Here's how the part is built. I have some questions about the finished solid (model axes, mm). A direction names the side the tool comes from. Round coordinates to 2 decimals unless told otherwise and drop trailing zeros. Write each loop counter-clockwise with the first axis right and the second up, starting at its lowest first coordinate (ties: lowest second). Pieces come first, ordered by that corner, then holes. Notation, with made-up numbers: (-10.5, -10.5) -> (32.5, -10.5) arc R16 cw to (32.5, -3.5) -> close; hole circle Ø6 at (16, 36.25). An arc over 180 degrees is marked (long way). Answer in a Markdown table with one row per item.
from build123d import *

# Parameters (mm, degrees)
F1_DEPTH     = 38.1
F3_DEPTH     = 38.1
F5_D         = 6.35
F6_T1_DEPTH  = 20.7437886812
F6_T3_DEPTH  = 27.94
F6_T5_DEPTH  = 49.7055689591
F6_T7_DEPTH  = 20.4179452734
F6_T9_DEPTH  = 49.0300859467
F6_T11_DEPTH = 71.8058781858
F6_T13_DEPTH = 25.3882661408
F6_T15_DEPTH = 70.8375780274
F6_T17_DEPTH = 26.1528668654
F6_T22_DEPTH = 5.08
F6_T28_DEPTH = 5.08
F6_T34_DEPTH = 5.08
F6_T40_DEPTH = 5.08


# Not quite as in the source:
# - a fillet or chamfer that OpenCascade refuses, or shapes differently, is made with other operations: its cross-section is extruded or revolved along the edge and cut away or added


with BuildPart() as f1:
    # F0 (on Front) → F1 (new body)
    with BuildSketch(Plane.XZ):
        Polygon((0, 38.1), (0, 0.2683098665), (38.1, 0), (38.1, 38.1), align=None)
    extrude(amount=F1_DEPTH)

    # F2 (on face) → F3 (cut)
    with BuildSketch(Plane.XZ.offset(38.1)):
        Polygon((29.289287496, 38.1), (6.7755630988, 38.1), (19.05, 25.849385187), align=None)
        Polygon((0, 38.1), (0, 25.849385187), (6.7755630988, 38.1), align=None)
        Polygon((29.289287496, 38.1), (38.1, 25.849385187), (38.1, 38.1), align=None)
        Polygon((0, 0.2683098665), (18.8937886297, 0.1352550134), (0, 16.4943691343), align=None)
        Polygon((38.1, 16.4943691343), (20.8069253196, 0.1217822194), (38.1, 0), align=None)
    extrude(amount=-F3_DEPTH, mode=Mode.SUBTRACT)

    # F5 (through all)
    with Locations(Plane.YZ.offset(38.1)):
        with Locations((-19.05, 21.1718771607)):
            Hole(F5_D / 2)

    # F6: fillet of radius 5.08 on 16 edges, made by hand

    # F6_s2 → F6_t1 (cut)
    with BuildSketch(Plane.XY.offset(3.7943691343)):
        with BuildLine():
            ThreePointArc((5.08, 0), (1.4878975516, -1.4878975516), (0, -5.08))
            Line((0, -5.08), (0, 0))
            Line((0, 0), (5.08, 0))
        make_face()
        with BuildLine():
            ThreePointArc((5.08, -38.1), (1.4878975516, -36.6121024484), (0, -33.02))
            Line((0, -33.02), (0, -38.1))
            Line((0, -38.1), (5.08, -38.1))
        make_face()
    extrude(amount=F6_T1_DEPTH, mode=Mode.SUBTRACT)

    # F6_s4 → F6_t3 (cut)
    with BuildSketch(Plane.XZ.offset(5.08)):
        with BuildLine():
            ThreePointArc((0.634616087, 26.9968082311), (0.1612120254, 25.8077738444), (0, 24.5381578155))
            Line((0, 24.5381578155), (0, 25.849385187))
            Line((0, 25.849385187), (0.634616087, 26.9968082311))
        make_face()
        with BuildLine():
            ThreePointArc((37.1441471446, 27.1784247107), (37.8551353391, 25.7704755844), (38.1, 24.2123144077))
            Line((38.1, 24.2123144077), (38.1, 25.849385187))
            Line((38.1, 25.849385187), (37.1441471446, 27.1784247107))
        make_face()
    extrude(amount=F6_T3_DEPTH, mode=Mode.SUBTRACT)

    # F6_s6 → F6_t5 (cut)
    with BuildSketch(Plane.XZ.offset(-5.8027844796)):
        with BuildLine():
            ThreePointArc((1.754752754, 14.9750232202), (0.4594666969, 16.704305057), (0, 18.8154829261))
            Line((0, 18.8154829261), (0, 16.4943691343))
            Line((0, 16.4943691343), (1.754752754, 14.9750232202))
        make_face()
    extrude(amount=F6_T5_DEPTH, mode=Mode.SUBTRACT)

    # F6_s8 → F6_t7 (cut)
    with BuildSketch(Plane.XY.offset(3.7943691343)):
        with BuildLine():
            ThreePointArc((33.02, 0), (36.6121024484, -1.4878975516), (38.1, -5.08))
            Line((38.1, -5.08), (38.1, 0))
            Line((38.1, 0), (33.02, 0))
        make_face()
        with BuildLine():
            ThreePointArc((33.02, -38.1), (36.6121024484, -36.6121024484), (38.1, -33.02))
            Line((38.1, -33.02), (38.1, -38.1))
            Line((38.1, -38.1), (33.02, -38.1))
        make_face()
    extrude(amount=F6_T7_DEPTH, mode=Mode.SUBTRACT)

    # F6_s10 → F6_t9 (cut)
    with BuildSketch(Plane.XZ.offset(-5.4650429733)):
        with BuildLine():
            ThreePointArc((38.1, 18.6803863236), (37.6863002203, 16.6723917386), (36.5125817899, 14.991447121))
            Line((36.5125817899, 14.991447121), (38.1, 16.4943691343))
            Line((38.1, 16.4943691343), (38.1, 18.6803863236))
        make_face()
    extrude(amount=F6_T9_DEPTH, mode=Mode.SUBTRACT)

    # F6_s12 → F6_t11 (cut)
    with BuildSketch(Plane.XZ.offset(-16.8529390929)):
        with BuildLine():
            ThreePointArc((11.5469219559, 33.3379013421), (7.2465010014, 34.7721948924), (3.5129264291, 32.2009618637))
            Line((3.5129264291, 32.2009618637), (6.7755630988, 38.1))
            Line((6.7755630988, 38.1), (11.5469219559, 33.3379013421))
        make_face()
    extrude(amount=F6_T11_DEPTH, mode=Mode.SUBTRACT)

    # F6_s14 → F6_t13 (cut)
    with BuildSketch(Plane(origin=(11.5824663758, 0, 20.9417773971), x_dir=(0, 1, 0), z_dir=(0.4839863023, 0, 0.8750755734))):
        with BuildLine():
            ThreePointArc((-38.1, 7.4307483528), (-36.6121024484, 11.0228508012), (-33.02, 12.5107483528))
            Line((-33.02, 12.5107483528), (-38.1, 12.5107483528))
            Line((-38.1, 12.5107483528), (-38.1, 7.4307483528))
        make_face()
        with BuildLine():
            ThreePointArc((0, 7.4307483528), (-1.4878975516, 11.0228508012), (-5.08, 12.5107483528))
            Line((-5.08, 12.5107483528), (0, 12.5107483528))
            Line((0, 12.5107483528), (0, 7.4307483528))
        make_face()
    extrude(amount=F6_T13_DEPTH, mode=Mode.SUBTRACT)

    # F6_s16 → F6_t15 (cut)
    with BuildSketch(Plane.XZ.offset(-16.3687890137)):
        with BuildLine():
            ThreePointArc((25.0903071925, 33.076204123), (29.1727291737, 34.8949986115), (33.1122507828, 32.7844650022))
            Line((33.1122507828, 32.7844650022), (29.289287496, 38.1))
            Line((29.289287496, 38.1), (25.0903071925, 33.076204123))
        make_face()
    extrude(amount=F6_T15_DEPTH, mode=Mode.SUBTRACT)

    # F6_s18 → F6_t17 (cut)
    with BuildSketch(Plane(origin=(-15.4901461094, 0, 21.5378510306), x_dir=(0, 1, 0), z_dir=(0.5838799809, 0, -0.8118399891))):
        with BuildLine():
            ThreePointArc((-33.02, 46.024042114), (-36.6121024484, 44.5361445625), (-38.1, 40.944042114))
            Line((-38.1, 40.944042114), (-38.1, 46.024042114))
            Line((-38.1, 46.024042114), (-33.02, 46.024042114))
        make_face()
        with BuildLine():
            ThreePointArc((-5.08, 46.024042114), (-1.4878975516, 44.5361445625), (0, 40.944042114))
            Line((0, 40.944042114), (0, 46.024042114))
            Line((0, 46.024042114), (-5.08, 46.024042114))
        make_face()
    extrude(amount=F6_T17_DEPTH, mode=Mode.SUBTRACT)


with BuildPart() as f6_tool20:
    # F6_s21 → F6_t22 (new body)
    with BuildSketch(Plane.XZ.offset(5.08)):
        Polygon((5.08, 24.5381578155), (0.634616087, 26.9968082311), (0, 25.849385187), (0, 24.5381578155), align=None)
    extrude(amount=-F6_T22_DEPTH)

    # F6_s23 → F6_t24 (revolve, cut)
    with BuildSketch(Plane(origin=(5.08, -5.08, 24.5381578155), x_dir=(0.9682653493, 0, -0.2499244151), z_dir=(0.2499244151, 0, 0.9682653493))):
        with BuildLine():
            ThreePointArc((0, -5.08), (5.08, 0), (0, 5.08))
            Line((0, 5.08), (0, -5.08))
        make_face()
    revolve(axis=Axis((5.08, -5.08, 24.5381578155), (0, 1, 0)), mode=Mode.SUBTRACT)


with BuildPart() as f1_1:
    add(f1.part)

    # F6_t19: cut F6_tool20
    add(f6_tool20.part, mode=Mode.SUBTRACT)


with BuildPart() as f6_tool26:
    # F6_s27 → F6_t28 (new body)
    with BuildSketch(Plane.XZ.offset(33.02)):
        Polygon((5.08, 24.5381578155), (0.634616087, 26.9968082311), (0, 25.849385187), (0, 24.5381578155), align=None)
    extrude(amount=F6_T28_DEPTH)

    # F6_s29 → F6_t30 (revolve, cut)
    with BuildSketch(Plane(origin=(5.08, -33.02, 24.5381578155), x_dir=(0.9682653493, 0, -0.2499244151), z_dir=(-0.2499244151, 0, -0.9682653493))):
        with BuildLine():
            ThreePointArc((0, -5.08), (5.08, 0), (0, 5.08))
            Line((0, 5.08), (0, -5.08))
        make_face()
    revolve(axis=Axis((5.08, -33.02, 24.5381578155), (0, -1, 0)), mode=Mode.SUBTRACT)


with BuildPart() as f1_2:
    add(f1_1.part)

    # F6_t25: cut F6_tool26
    add(f6_tool26.part, mode=Mode.SUBTRACT)


with BuildPart() as f6_tool32:
    # F6_s33 → F6_t34 (new body)
    with BuildSketch(Plane.XZ.offset(5.08)):
        Polygon((33.02, 24.2123144077), (38.1, 24.2123144077), (38.1, 25.849385187), (37.1441471446, 27.1784247107), align=None)
    extrude(amount=-F6_T34_DEPTH)

    # F6_s35 → F6_t36 (revolve, cut)
    with BuildSketch(Plane(origin=(33.02, -5.08, 24.2123144077), x_dir=(-0.9517982951, 0, -0.3067246411), z_dir=(0.3067246411, 0, -0.9517982951))):
        with BuildLine():
            ThreePointArc((0, -5.08), (5.08, 0), (0, 5.08))
            Line((0, 5.08), (0, -5.08))
        make_face()
    revolve(axis=Axis((33.02, -5.08, 24.2123144077), (0, 1, 0)), mode=Mode.SUBTRACT)


with BuildPart() as f1_3:
    add(f1_2.part)

    # F6_t31: cut F6_tool32
    add(f6_tool32.part, mode=Mode.SUBTRACT)


with BuildPart() as f6_tool38:
    # F6_s39 → F6_t40 (new body)
    with BuildSketch(Plane.XZ.offset(33.02)):
        Polygon((33.02, 24.2123144077), (38.1, 24.2123144077), (38.1, 25.849385187), (37.1441471446, 27.1784247107), align=None)
    extrude(amount=F6_T40_DEPTH)

    # F6_s41 → F6_t42 (revolve, cut)
    with BuildSketch(Plane(origin=(33.02, -33.02, 24.2123144077), x_dir=(-0.9517982951, 0, -0.3067246411), z_dir=(-0.3067246411, 0, 0.9517982951))):
        with BuildLine():
            ThreePointArc((0, -5.08), (5.08, 0), (0, 5.08))
            Line((0, 5.08), (0, -5.08))
        make_face()
    revolve(axis=Axis((33.02, -33.02, 24.2123144077), (0, -1, 0)), mode=Mode.SUBTRACT)


with BuildPart() as f1_4:
    add(f1_3.part)

    # F6_t37: cut F6_tool38
    add(f6_tool38.part, mode=Mode.SUBTRACT)

    # F6_s43 → F6_t44 (revolve, cut)
    with BuildSketch(Plane.XY.offset(21.1718771607)):
        with BuildLine():
            ThreePointArc((0, -10.795), (1.4878975516, -14.3871024484), (5.08, -15.875))
            Line((5.08, -15.875), (0, -15.875))
            Line((0, -15.875), (0, -10.795))
        make_face()
    revolve(axis=Axis((0, -19.05, 21.1718771607), (1, 0, 0)), mode=Mode.SUBTRACT)

    # F6_s45 → F6_t46 (revolve, cut)
    with BuildSketch(Plane.XY.offset(21.1718771607)):
        with BuildLine():
            ThreePointArc((38.1, -10.795), (36.6121024484, -14.3871024484), (33.02, -15.875))
            Line((33.02, -15.875), (38.1, -15.875))
            Line((38.1, -15.875), (38.1, -10.795))
        make_face()
    revolve(axis=Axis((38.1, -19.05, 21.1718771607), (1, 0, 0)), mode=Mode.SUBTRACT)


solid = f1_4.part
1) I want a section at D-D, the plane x = 21.5. List the corners of the cut face in (y, z) for me (3 decimals), and give its area (3 significant figures).
Response:
| item | result |
|---|---|
| outline | (-38.1, 0.778) -> (0, 0.778) -> (0, 28.781) -> (-38.1, 28.781) -> close; hole circle Ø6.35 at (-19.05, 21.172) |
| area | 1,040 mm^2 |
2) Which directions (+Z, -Z, +X, -X, +Y, -Y) give clear straight access to the entire face, cutting with the end or side of a thin tool? Please do faces 1 (the face through (22.028, -19.317, 29.412)), 2 (the face through (18.85, -16.53, 19.24)).
Response:
| item | result |
|---|---|
| face 1 | +Z, +Y, -Y |
| face 2 | +X, -X |
3) I want a section at B-B, the plane x = 13.5. List the corners of the cut face in (y, z) for me (3 decimals).
Response:
| item | result |
|---|---|
| outline | (-38.1, 4.805) -> (0, 4.805) -> (0, 31.389) -> (-38.1, 31.389) -> close; hole circle Ø6.35 at (-19.05, 21.172) |
4) I need wall thicknesses on line 1 (Z direction, x = 20, y = -19); line 2 (X direction, y = -10, z = 30); line 3 (X direction, y = -18.5, z = 27). Which ranges of each line are inside material? Lowest first, please. Write a range as [from, to].
Response:
| item | result |
|---|---|
| line 1 | z = [0.13, 18], [24.35, 26.99] |
| line 2 | x = [2.3, 14.89], [22.52, 35.11] |
| line 3 | x = [0.64, 17.9], [20.01, 37.27] |
5) We'd pull the mould along X, two halves only. Please class faces 3 (the face through (28.77, -19.32, 7.66)), 4 (the face through (7.31, -18.78, 34.78)), 5 (the face through (19, 0, 17)), 6 (the face through (29.108, -18.783, 34.897)): +X half, -X half, draft (parallel to the pull), parting line (faces both ways), or undercut.
Response:
| item | result |
|---|---|
| face 3 | +X half |
| face 4 | undercut |
| face 5 | draft |
| face 6 | undercut |
6) For pin 1 (1 mm diameter, centred on x = 24, y = -19.5, fed in from +Z); pin 2 (2 mm diameter, centred on x = 32.5, y = -15, fed in from +Z); pin 3 (4 mm diameter, centred on y = -19.05, z = 21.17, fed in from -X); pin 4 (3 mm diameter, centred on y = -5.5, z = 7, fed in from -X), each with a flat end and sliding along its axis, tell me the tip position at first contact or that it passes through.
Response:
| item | result |
|---|---|
| pin 1 | stops at z = 32.37 |
| pin 2 | stops at z = 34.23 |
| pin 3 | passes through |
| pin 4 | stops at x = 9.23 |
7) I want a section at C-C, the plane y = -4. List the corners of the cut face in (x, z) for me.
Response:
| item | result |
|---|---|
| outline | (0.12, 17.74) arc R5.08 ccw to (1.75, 14.98) -> (18.89, 0.14) -> (20.81, 0.12) -> (36.51, 14.99) arc R5.08 ccw to (37.98, 17.6) -> (37.98, 24.21) arc R4.96 ccw to (37.05, 27.11) -> (32.39, 33.59) arc R5.08 ccw to (25.09, 33.08) -> (19.05, 25.85) -> (11.55, 33.34) arc R5.08 ccw to (4.14, 33.09) -> (0.74, 26.94) arc R4.96 ccw to (0.12, 24.54) -> close |
